from build123d import *

# Parameters (mm, degrees)
SKETCH063_W   = 6.3
SKETCH063_H   = 9.3
PAD029_DEPTH  = 5
SKETCH064_R   = 2.75
PAD030_DEPTH  = 3
CHAMFER_SIZE2 = 5
CHAMFER_SIZE  = 15


with BuildPart() as part:
    # Sketch063 → Pad029 (new body)
    with BuildSketch(Plane.XY):
        with BuildLine():
            Line((-6.15, 4.65), (-6.15, -4.65))
            ThreePointArc((-6.15, -4.65), (-5.2713203436, -6.7713203436), (-3.15, -7.65))
            Line((-3.15, -7.65), (38.5, -7.65))
            Line((38.5, -7.65), (38.5, 7.65))
            Line((38.5, 7.65), (-3.15, 7.65))
            ThreePointArc((-3.15, 7.65), (-5.2713203436, 6.7713203436), (-6.15, 4.65))
        make_face()
        Rectangle(SKETCH063_W, SKETCH063_H, mode=Mode.SUBTRACT)
    extrude(amount=PAD029_DEPTH)

    # Sketch064 (on Face4 of Pad029) → Pad030 (join)
    with BuildSketch(Plane.YZ.offset(38.5)):
        with BuildLine():
            Line((-7.65, 19), (-7.65, 5))
            Line((-7.65, 5), (7.65, 5))
            Line((7.65, 5), (7.65, 19))
            ThreePointArc((7.65, 19), (6.7713203436, 21.1213203436), (4.65, 22))
            Line((4.65, 22), (-4.65, 22))
            ThreePointArc((-4.65, 22), (-6.7713203436, 21.1213203436), (-7.65, 19))
        make_face()
        with Locations((0, 16)):
            Circle(SKETCH064_R, mode=Mode.SUBTRACT)
    extrude(amount=-PAD030_DEPTH)

    # Chamfer
    chamfer_edges = [part.edges().sort_by_distance(p)[0] for p in [
        (35.5, 0, 5),
    ]]
    chamfer_side = part.faces().sort_by_distance((16.306308, 0, 5))[0]
    chamfer(chamfer_edges, length=CHAMFER_SIZE, length2=CHAMFER_SIZE2, reference=chamfer_side)


with BuildPart() as part_1:
    # Body017 placement: moved
    add(part.part.moved(Location((3, -2.563e-05, 214))))


solid = part_1.part
Geometry check sheet. Reference: the model listing, model coordinates, mm. A direction names the side the tool comes from. Round coordinates to 2 decimals unless told otherwise and drop trailing zeros. Order: outer loops, then holes, each group sorted by start corner. A loop starts at its lowest first (then second) coordinate and runs counter-clockwise, first axis right, second up. Notation, with made-up numbers: M 53,-31 L 74,-31 A16 cw 74,-9 Z; hole C 10,68.25 d9. An arc over 180 degrees is marked long. Write each question's results on one line, items separated by ' | '. Start each with the question number.
1. Material ranges on L1, parallel to Y at x = 40, z = 230; L2, parallel to X at y = -3.25, z = 216; L3, parallel to Z at x = -0.5, y = 4, recorded low to high. Write a range as from..to.
2. Set-up check for faces 1 (the face through (6.15, 0, 216)), 2 (the face through (38.5, 0, 233)), 3 (the face through (41.5, 0, 225)): record each of +Z, -Z, +X, -X, +Y, -Y from which the full face is reachable in a straight line by a thin tool's end or side.
3. Go/stop test with flat-tipped pins: P1, Ø6, axis at x = 2, y = -4.5, coming from the +Z side; P2, Ø2, axis at y = -1, z = 232.5, coming from the -X side; P3, Ø1.5, axis at x = 32.5, y = 1.5, coming from the +Z side. Record where each tip stops, or that it passes through.
4. Cross-section at C-C on z = 218.25. Record the boundary of the cut face in (x, y).
5. Cross-section at B-B on y = -3.25. Record the boundary of the cut face in (x, z), plus the area to 3 significant figures.
6. Cross-section at D-D on z = 230. Record the boundary of the cut face in (x, y), plus the area to 3 significant figures.
7. Draft check along X on faces 4 (the face through (25, -7.65, 219)), 5 (the face through (3, 4.65, 216)), 6 (the face through (31.105, -0.107, 221.535)). Enter one of: pulls with the +X half, pulls with the -X half, needs draft (parallel to the pull), parting line crosses it, or undercut.
8. Cross-section at A-A on x = 4. Record the boundary of the cut face in (y, z), plus the area to 3 significant figures.
Resolved:
1) L1: -7.65..-2.75, 2.75..7.65 | L2: -3.15..-0.15, 6.15..41.5 | L3: 214..219
2) face 1: +Z, -Z | face 2: +Z, -X, +Y, -Y | face 3: +Z, -Z, +X, +Y, -Y
3) P1: z = 219 | P2: x = 38.5 | P3: z = 222.25
4) outline: M -3.15,-4.65 A3 ccw -0.15,-7.65 L 41.5,-7.65 L 41.5,7.65 L -0.15,7.65 A3 ccw -3.15,4.65 Z; hole M -0.15,-4.65 L 6.15,-4.65 L 6.15,4.65 L -0.15,4.65 Z
5) outline: M -3.15,214 L -0.15,214 L -0.15,219 L -3.15,219 Z; M 6.15,214 L 41.5,214 L 41.5,236 L 38.5,236 L 38.5,224 L 23.5,219 L 6.15,219 Z | area: 280 mm2
6) outline: M 38.5,-7.65 L 41.5,-7.65 L 41.5,-2.75 L 38.5,-2.75 Z; M 38.5,2.75 L 41.5,2.75 L 41.5,7.65 L 38.5,7.65 Z | area: 29.4 mm2
7) face 4: needs draft | face 5: undercut | face 6: pulls with the -X half
8) outline: M -7.65,214 L -4.65,214 L -4.65,219 L -7.65,219 Z; M 4.65,214 L 7.65,214 L 7.65,219 L 4.65,219 Z | area: 30.0 mm2
